from build123d import *

# Parameters (mm, degrees)
BOSS_EXTRU_1_DEPTH = 80
COQUE1_START       = 4
COQUE1_DEPTH       = 72
CONG_1_R           = 2


# Read off the part's stored shape, not the designer's step: Coque1
with BuildPart() as part:
    # Esquisse1 → Boss.-Extru.1 (new body)
    with BuildSketch(Plane.XY):
        Polygon((-590, 1310.680153009), (-590, 440.370234654), (-344.477435621, -40), (344.477435621, -40), (590, 440.370234654), (590, 1310.680153009), (343.14108798, 1740), (-343.14108798, 1740), align=None)
        Polygon((-320, 1700), (320, 1700), (550, 1300), (550, 450), (320, 0), (-320, 0), (-550, 450), (-550, 1300), align=None, mode=Mode.SUBTRACT)
    extrude(amount=BOSS_EXTRU_1_DEPTH)

    # Coque1 outline → Coque1 (cut)
    with BuildSketch(Plane.XY.offset(COQUE1_START)):
        Polygon((-340.826979182, 1736), (-586, 1309.612137708), (-586, 441.333211189), (-342.029692059, -36), (342.029692059, -36), (586, 441.333211189), (586, 1309.612137708), (340.826979182, 1736), align=None)
        Polygon((-554, 449.037023465), (-554, 1301.068015301), (-322.314108798, 1704), (322.314108798, 1704), (554, 1301.068015301), (554, 449.037023465), (322.447743562, -4), (-322.447743562, -4), align=None, mode=Mode.SUBTRACT)
    extrude(amount=COQUE1_DEPTH, mode=Mode.SUBTRACT)

    # Congé1
    cong_1_edges = [part.edges().sort_by_distance(p)[0] for p in [
        (-467.238717811, 200.185117327, 80),
        (-590, 875.525193832, 0),
        (-466.57054399, 1525.340076505, 0),
        (0, -40, 80),
        (467.238717811, 200.185117327, 80),
        (590, 875.525193832, 80),
        (466.57054399, 1525.340076505, 80),
        (0, 1740, 80),
        (-435, 1500, 0),
        (-550, 875, 0),
        (-435, 225, 0),
        (0, 0, 0),
        (435, 225, 0),
        (550, 875, 0),
        (435, 1500, 0),
        (0, 1700, 0),
        (-435, 1500, 80),
        (-550, 875, 80),
        (-435, 225, 80),
        (0, 0, 80),
        (435, 225, 80),
        (550, 875, 80),
        (435, 1500, 80),
        (0, 1700, 80),
        (-466.57054399, 1525.340076505, 80),
        (-463.413489591, 1522.806068854, 76),
        (-586, 875.472674449, 76),
        (-464.01484603, 202.666605594, 76),
        (0, -36, 76),
        (464.01484603, 202.666605594, 76),
        (586, 875.472674449, 76),
        (463.413489591, 1522.806068854, 76),
        (0, 1736, 76),
        (0, 1704, 4),
        (-438.157054399, 1502.53400765, 4),
        (-554, 875.052519383, 4),
        (-438.223871781, 222.518511733, 4),
        (0, -4, 4),
        (438.223871781, 222.518511733, 4),
        (554, 875.052519383, 4),
        (438.157054399, 1502.53400765, 4),
        (-463.413489591, 1522.806068854, 4),
        (-586, 875.472674449, 4),
        (-464.01484603, 202.666605594, 4),
        (0, -36, 4),
        (464.01484603, 202.666605594, 4),
        (586, 875.472674449, 4),
        (463.413489591, 1522.806068854, 4),
        (0, 1736, 4),
        (-438.157054399, 1502.53400765, 76),
        (-554, 875.052519383, 76),
        (-438.223871781, 222.518511733, 76),
        (0, -4, 76),
        (438.223871781, 222.518511733, 76),
        (554, 875.052519383, 76),
        (438.157054399, 1502.53400765, 76),
        (0, 1704, 76),
        (-590, 875.525193832, 80),
        (0, 1740, 0),
        (466.57054399, 1525.340076505, 0),
        (590, 875.525193832, 0),
        (467.238717811, 200.185117327, 0),
        (0, -40, 0),
        (-467.238717811, 200.185117327, 0),
    ]]
    fillet(cong_1_edges, radius=CONG_1_R)


solid = part.part
Read the model definition and answer for the solid it produces. Units are mm, in the model's axes. A direction names the side the tool comes from. Round coordinates to 2 decimals unless told otherwise and drop trailing zeros. Use one line per item in the form item = value. Start each with the question number.
(1) Determine the mould class of faces 5 (the face through (-468.96, 203.55, 39.47)), 6 (the face through (464.32, 1528.05, 79.43)), 7 (the face through (433.751, 221.235, 79.43)), 8 (the face through (-440.22, 225.1, 4.57)) for opening direction X: +X half, -X half, draft (parallel to the pull), parting line (faces both ways), or undercut.
(2) For faces 1 (the face through (-467.8, 1522.05, 0.6)), 2 (the face through (433.39, 1502.8, 39.47)), 3 (the face through (-433.75, 1503.38, 79.43)), 4 (the face through (586, 869, 40)), determine the directions among +Z, -Z, +X, -X, +Y, -Y from which every point of the face is accessible in a straight line to the end or side of a thin tool.
(3) The part is cut by section A-A (y = 949). Count the separate pieces of the cut face and the enclosed holes in it, then the cut area to 3 significant figures.
(4) Find the intervals of material crossed by line 1 along Y through (x, z) = (-188, 61.5); line 2 along X through (y, z) = (1070, 27.5); line 3 along X through (y, z) = (673, 74.5), in increasing order. Write a range as from..to.
Checked values:
q1.face_5 = -X half
q1.face_6 = +X half
q1.face_7 = undercut
q1.face_8 = undercut
q2.face_1 = -Z, -X, +Y
q2.face_2 = +Z, -Z
q2.face_3 = +Z
q2.face_4 = none
q3.separate_pieces = 2
q3.enclosed_holes = 2
q3.area = 1,790 mm^2
q4.line_1 = -40..-36, -4..0, 1700..1704, 1736..1740
q4.line_2 = -590..-586, -554..-550, 550..554, 586..590
q4.line_3 = -590..-585.94, -554.06..-550, 550..554.06, 585.94..590
